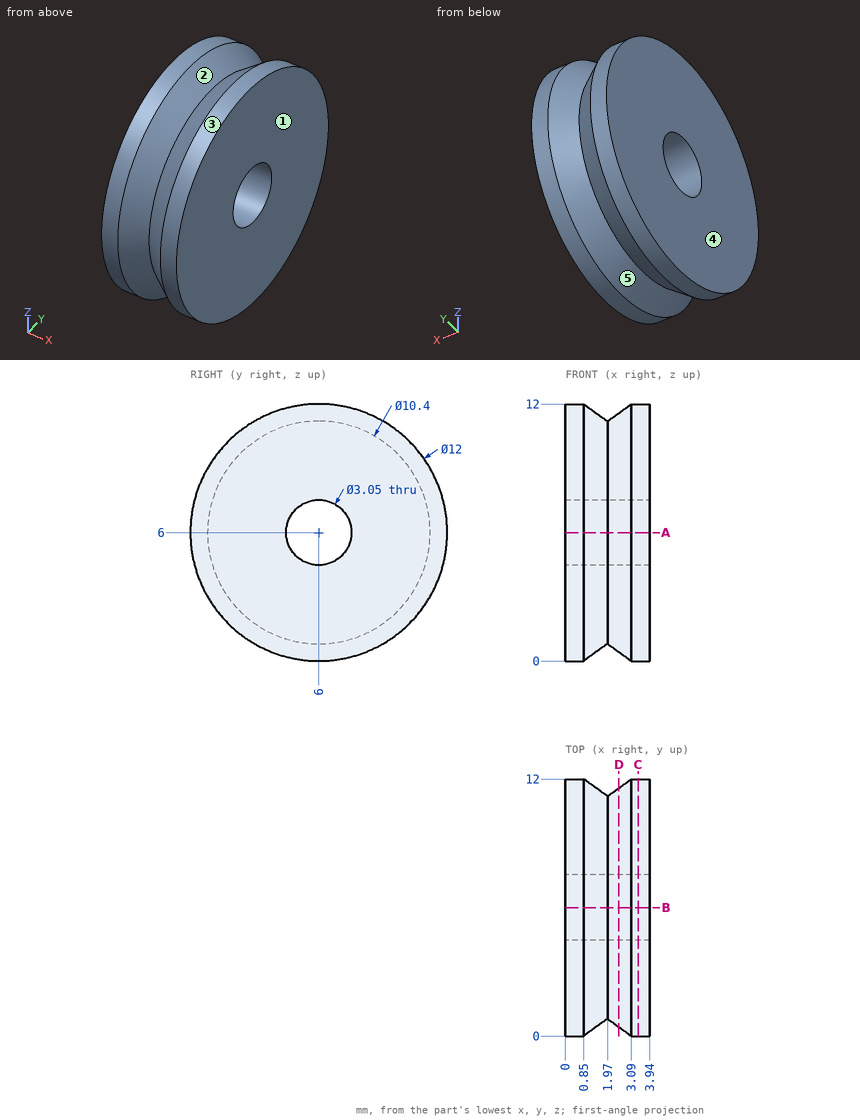
Geometry check sheet. Reference: drawing and pictorial views, mm from the part's lowest x, y, z. A direction names the side the tool comes from. Coordinates: 2 decimals unless noted, no trailing zeros. Order: outer loops, then holes, each group sorted by start corner. A loop starts at its lowest first (then second) coordinate and runs counter-clockwise, first axis right, second up.
Item 1: Depth check by flat-ended pin: pin 1 (1.5 mm diameter, centred on x = 1, y = 4.5, fed in from +Z); pin 2 (1 mm diameter, centred on x = 3, y = 3, fed in from +Z); pin 3 (1 mm diameter, centred on x = 0.5, z = 10, fed in from -Y). Enter the tip coordinate at first touch or a pass-through.
Item 2: Section check A-A (z = 6). Enter the section's corners in (x, y) (3 decimals).
Item 3: Mould release check, pull along X, two halves, no side actions. Record for the marked faces 3, 4 and 5: released by +X, released by -X, zero draft, split by the parting line, or undercut.
Item 4: Tool access check on the marked faces 1 and 2. Record the directions out of +Z, -Z, +X, -X, +Y, -Y that give a thin tool (end or side, any length) a straight path to the whole face; none if there is none.
Item 5: Scan lines: line 1 along Y through (x, z) = (3.15, 6) (3 decimals); line 2 along X through (y, z) = (10.5, 2.75); line 3 along Y through (x, z) = (1.3, 6) (3 decimals). Record each from-to range of solid material in increasing order.
Item 6: Section check C-C (x = 3.4). Enter the section's corners in (y, z) (3 decimals), plus the area to 3 significant figures.
Item 7: Section check D-D (x = 2.5). Enter the section's corners in (y, z) (3 decimals).
Check sheet entries:
1. pin 1: stops at z = 11.95
1. pin 2: stops at z = 11.45
1. pin 3: stops at y = 1.13
2. outline: (0, 0) - (0.85, 0) - (1.97, 0.8) - (3.09, 0) - (3.94, 0) - (3.94, 4.475) - (0, 4.475) - close; (0, 7.525) - (3.94, 7.525) - (3.94, 12) - (3.09, 12) - (1.97, 11.2) - (0.85, 12) - (0, 12) - close
3. face 3: zero draft
3. face 4: released by -X
3. face 5: undercut
4. face 1: +Z, -Z, +X, +Y, -Y
4. face 2: none
5. line 1: y = 0 to 4.475, 7.525 to 12
5. line 2: x = 0 to 1.48, 2.46 to 3.94
5. line 3: y = 0.321 to 4.475, 7.525 to 11.679
6. outline: circle Ø12 at (6, 6); hole circle Ø3.05 at (6, 6)
6. area: 106 mm2
7. outline: circle Ø11.157 at (6, 6); hole circle Ø3.05 at (6, 6)
